CAD build for the part. Positions are in the model's coordinates, mm. Face numbers are marked on the shaded views. Coordinates: 2 decimals unless noted, no trailing zeros. Write each loop counter-clockwise with the first axis right and the second up, starting at its lowest first coordinate (ties: lowest second). Pieces come first, ordered by that corner, then holes.
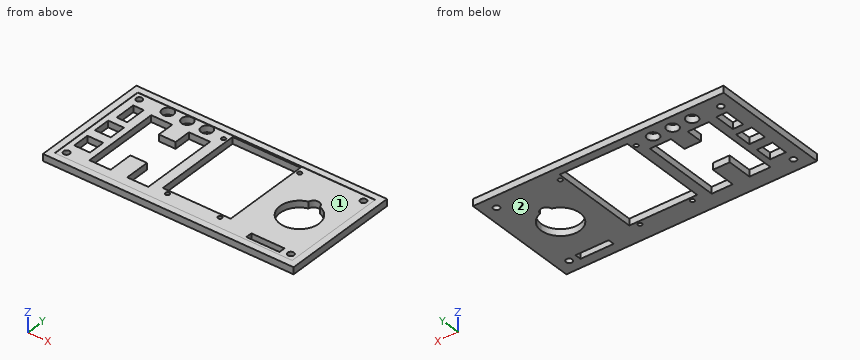
```python
from build123d import *

# Parameters (mm, degrees)
MODEL_W             = 114.2864
MODEL_H             = 50.7864
MODEL_R             = 1.5
MODEL_W_2           = 7.5932
MODEL_H_2           = 8.1012
MODEL_R_2           = 1
MODEL_W_3           = 15.9766
MODEL_H_3           = 3.0734
MODEL_W_4           = 5.0528
MODEL_H_4           = 10.132799902
MODEL_R_3           = 2.7813
MODEL_W_5           = 32.6908
MODEL_H_5           = 42.6908
BOSS_EXTRUDE1_DEPTH = 3.175
SKETCH1_W           = 120.636394244
SKETCH1_H           = 57.136394614
SKETCH1_W_2         = 114.2864
SKETCH1_H_2         = 50.7864
BOSS_EXTRUDE2_DEPTH = 3.302


with BuildPart() as part:
    # Model → Boss-Extrude1 (new body)
    with BuildSketch(Plane.XY):
        with Locations((57.143197122, 25.393197307)):
            Rectangle(MODEL_W, MODEL_H)
        with Locations((3.175, 3.175)):
            Circle(MODEL_R, mode=Mode.SUBTRACT)
        with Locations((6.343197122, 12.693197307)):
            Rectangle(MODEL_W_2, MODEL_H_2, mode=Mode.SUBTRACT)
        with Locations((49.9364, 5.5118)):
            Circle(MODEL_R_2, mode=Mode.SUBTRACT)
        with Locations((6.343197122, 25.393197307)):
            Rectangle(MODEL_W_2, MODEL_H_2, mode=Mode.SUBTRACT)
        Polygon((23.272097122, 4.543497307), (13.137897122, 4.543497307), (13.137897122, 42.280497307), (23.272097122, 42.280497307), (23.272097122, 34.120497307), (31.314978679, 34.120497307), (31.314978679, 42.301497307), (41.449178679, 42.301497307), (41.449178679, 4.522497307), (31.314978679, 4.522497307), (31.314978679, 16.629297307), (23.272097122, 16.629297307), align=None, mode=Mode.SUBTRACT)
        with Locations((75.184, 5.5118)):
            Circle(MODEL_R_2, mode=Mode.SUBTRACT)
        with Locations((98.979297122, 3.0734)):
            Rectangle(MODEL_W_3, MODEL_H_3, mode=Mode.SUBTRACT)
        with Locations((111.125, 3.175)):
            Circle(MODEL_R, mode=Mode.SUBTRACT)
        with Locations((6.343197122, 38.093197307)):
            Rectangle(MODEL_W_4, MODEL_H_4, mode=Mode.SUBTRACT)
        with Locations((3.175, 47.625)):
            Circle(MODEL_R, mode=Mode.SUBTRACT)
        with Locations((16.764, 47.879)):
            Circle(MODEL_R_3, mode=Mode.SUBTRACT)
        with Locations((26.162, 47.879)):
            Circle(MODEL_R_3, mode=Mode.SUBTRACT)
        with Locations((35.56, 47.879)):
            Circle(MODEL_R_3, mode=Mode.SUBTRACT)
        with Locations((44.2722, 47.0662)):
            Circle(MODEL_R_2, mode=Mode.SUBTRACT)
        with Locations((62.553997122, 28.695197307)):
            Rectangle(MODEL_W_5, MODEL_H_5, mode=Mode.SUBTRACT)
        with BuildLine():
            ThreePointArc((100.60678971, 34.352628207), (105.35704277, 30.951911366), (107.1753, 25.4))
            ThreePointArc((107.1753, 25.4), (92.170948878, 17.88267863), (95.133038042, 34.401355967))
            ThreePointArc((95.133038042, 34.401355967), (97.890845314, 36.728290305), (100.60678971, 34.352628207))
        make_face(mode=Mode.SUBTRACT)
        with Locations((80.8482, 47.0662)):
            Circle(MODEL_R_2, mode=Mode.SUBTRACT)
        with Locations((111.125, 47.625)):
            Circle(MODEL_R, mode=Mode.SUBTRACT)
    extrude(amount=BOSS_EXTRUDE1_DEPTH)

    # Sketch1 → Boss-Extrude2 (add)
    with BuildSketch(Plane.XY):
        with Locations((57.143197122, 25.393197307)):
            Rectangle(SKETCH1_W, SKETCH1_H)
        with Locations((57.143197122, 25.393197307)):
            Rectangle(SKETCH1_W_2, SKETCH1_H_2, mode=Mode.SUBTRACT)
    extrude(amount=BOSS_EXTRUDE2_DEPTH)


solid = part.part
```
Item 1: Saw through at D-D, the plane x = 97.79. Write the cut outline in (y, z) (3 decimals), and give its area (3 significant figures).
Item 2: Flat gauge pins, fed straight in: pin 1 Ø3.5 at (x, y) = (111.125, 3.175) entering from -Z; pin 2 Ø1.8 at (x, y) = (80.85, 47.07) entering from +Z. Where does each tip first touch, or does it go through?
Item 3: Two-plate mould, pull along Y, no slides. Class the marked faces 1 and 2: +Y half, -Y half, draft (parallel to the pull), parting line (faces both ways), or undercut.
Item 4: Wall check: line 1 along X through (y, z) = (9, 1.35) (3 decimals); line 2 along X through (y, z) = (8, 0.85) (3 decimals); line 3 along Y through (x, z) = (50, 0.6) (3 decimals). Give the ranges that are in metal, low to high.
Item 5: Saw through at B-B, the plane x = 35.56. State how many separate pieces and enclosed holes the cut face has, and give its area (3 significant figures).
Item 6: Saw through at A-A, the plane y = 12.5. Write the cut outline in (x, z) (3 decimals), and give its area (3 significant figures).
Item 7: Saw through at C-C, the plane y = 41. Write the cut outline in (x, z) (3 decimals).
Working result:
1. outline: (-3.175, 0) - (1.537, 0) - (1.537, 3.175) - (0, 3.175) - (0, 3.302) - (-3.175, 3.302) - close; (4.61, 0) - (16.015, 0) - (16.015, 3.175) - (4.61, 3.175) - close; (36.727, 0) - (53.961, 0) - (53.961, 3.302) - (50.786, 3.302) - (50.786, 3.175) - (36.727, 3.175) - close
1. area: 107 mm2
2. pin 1: stops at z = 0
2. pin 2: passes through
3. face 1: undercut
3. face 2: draft
4. line 1: x = -3.175 to 2.547, 10.14 to 13.138, 23.272 to 31.315, 41.449 to 46.209, 78.899 to 117.461
4. line 2: x = -3.175 to 13.138, 23.272 to 31.315, 41.449 to 46.209, 78.899 to 117.461
4. line 3: y = -3.175 to 4.514, 6.51 to 7.35, 50.041 to 53.961
5. separate pieces: 3
5. enclosed holes: 0
5. area: 44.6 mm2
6. outline: (-3.175, 0) - (2.547, 0) - (2.547, 3.175) - (0, 3.175) - (0, 3.302) - (-3.175, 3.302) - close; (10.14, 0) - (13.138, 0) - (13.138, 3.175) - (10.14, 3.175) - close; (23.272, 0) - (31.315, 0) - (31.315, 3.175) - (23.272, 3.175) - close; (41.449, 0) - (46.209, 0) - (46.209, 3.175) - (41.449, 3.175) - close; (78.899, 0) - (117.461, 0) - (117.461, 3.302) - (114.286, 3.302) - (114.286, 3.175) - (78.899, 3.175) - close
6. area: 192 mm2
7. outline: (-3.175, 0) - (3.817, 0) - (3.817, 3.175) - (0, 3.175) - (0, 3.302) - (-3.175, 3.302) - close; (8.87, 0) - (13.138, 0) - (13.138, 3.175) - (8.87, 3.175) - close; (23.272, 0) - (31.315, 0) - (31.315, 3.175) - (23.272, 3.175) - close; (41.449, 0) - (46.209, 0) - (46.209, 3.175) - (41.449, 3.175) - close; (78.899, 0) - (117.461, 0) - (117.461, 3.302) - (114.286, 3.302) - (114.286, 3.175) - (78.899, 3.175) - close
